Work out the finished part from the listing and answer in its coordinate system (mm). A direction names the side the tool comes from. Round coordinates to 2 decimals unless told otherwise and drop trailing zeros. Loops run counter-clockwise (first coordinate to the right, second up) from the corner with the lowest first, then second, coordinate; pieces in that order, holes last. Notation, with made-up numbers: (-17.5, 61) -> (40.5, 61) arc R6 cw to (40.5, 66) -> close; hole circle Ø10 at (6, 41.25). An arc over 180 degrees is marked (long way). Use one line per item in the form item = value.
```python
from build123d import *

# Parameters (mm, degrees)
F0_R     = 10
F0_R_2   = 6.25
F1_DEPTH = 5
F0_R_3   = 5
F2_DEPTH = 55
F3_DEPTH = 51


# Not quite as in the source:
# - a fillet or chamfer that OpenCascade refuses, or shapes differently, is made with other operations: its cross-section is extruded or revolved along the edge and cut away or added


with BuildPart() as f1:
    # F0 (on Top) → F1 (new body)
    with BuildSketch(Plane.XY):
        Circle(F0_R)
        Circle(F0_R_2, mode=Mode.SUBTRACT)
    extrude(amount=F1_DEPTH)

    # F0 (on Top) → F2 (join)
    with BuildSketch(Plane.XY):
        Circle(F0_R_2)
        Circle(F0_R_3, mode=Mode.SUBTRACT)
    extrude(amount=F2_DEPTH)

    # F0 (on Top) → F3 (cut)
    with BuildSketch(Plane.XY):
        Circle(F0_R_3)
    extrude(amount=F3_DEPTH, mode=Mode.SUBTRACT)

    # F4: fillet of radius 2 on 3 edges, made by hand

    # F4_s1 → F4_t2 (revolve, cut)
    with BuildSketch(Plane.XZ):
        with BuildLine():
            ThreePointArc((5, 2), (5.5857864376, 0.5857864376), (7, 0))
            Line((7, 0), (5, 0))
            Line((5, 0), (5, 2))
        make_face()
    revolve(axis=Axis((0, 0, 0), (0, 0, 1)), mode=Mode.SUBTRACT)

    # F4_s3 → F4_t4 (revolve, cut)
    with BuildSketch(Plane.XZ):
        with BuildLine():
            ThreePointArc((6.25, 55), (5.3416876048, 54.263984367), (5, 53.1459503782))
            Line((5, 53.1459503782), (5, 55))
            Line((5, 55), (6.25, 55))
        make_face()
    revolve(axis=Axis((0, 0, 55), (0, 0, 1)), mode=Mode.SUBTRACT)

    # F4_s5 → F4_t6 (revolve, cut)
    with BuildSketch(Plane.XZ):
        with BuildLine():
            ThreePointArc((10, 2), (9.4142135624, 0.5857864376), (8, 0))
            Line((8, 0), (10, 0))
            Line((10, 0), (10, 2))
        make_face()
    revolve(axis=Axis((0, 0, 0), (0, 0, 1)), mode=Mode.SUBTRACT)


solid = f1.part
```
(1) For a pull along Y with two mould halves and no side action, classify faces 1 (the cylindrical face through (-1.08, -4.88, 27.21)), 2 (the cylindrical face through (5.96, 1.88, 29.65)), 3 (the flat face through (4, -6, 0)) as +Y half, -Y half, draft (parallel to the pull), parting line (faces both ways), or undercut.
Completed:
face_1 = undercut
face_2 = parting line
face_3 = draft
(2) Consider L1, parallel to Y at x = 0, z = 41; L2, parallel to Y at x = -3.5, z = 52; L3, parallel to Z at x = -7.5, y = 2. Determine where each line is inside the solid, lowest interval first.
Completed:
L1 = -6.25 to -5, 5 to 6.25
L2 = -5.18 to -3.57, 3.57 to 5.18
L3 = 0 to 5
(3) Given P1, Ø10, axis at y = 5, z = 24, coming from the -X side; P2, Ø8, axis at y = -3.5, z = 26.5, coming from the +X side; P3, Ø10, axis at x = -1.5, y = 0.5, coming from the +Z side; P4, Ø3, axis at x = 6.5, z = 47.5, coming from the +Y side, each flat-ended and moving along its own axis, determine where each tip first touches the part or whether it passes through.
Completed:
P1 = -6.25
P2 = 6.25
P3 = 55
P4 = 3.75
(4) For faces 4 (the flat face through (4, 5, 5)), 5 (the cylindrical face through (-2.17, -9.76, 3.48)), determine the directions among +Z, -Z, +X, -X, +Y, -Y from which every point of the face is accessible in a straight line to the end or side of a thin tool.
Completed:
face_4 = +Z
face_5 = +Z, -Z
(5) Find section A-A, the plane y = 0. Write down the section's boundary in (x, z), then the cut area to 3 significant figures.
Completed:
outline = (-10, 2) arc R2 ccw to (-8, 0) -> (-7, 0) arc R2 ccw to (-5, 2) -> (-5, 53.15) arc R2 ccw to (-6.25, 55) -> (-6.25, 5) -> (-10, 5) -> close; (5, 2) arc R2 ccw to (7, 0) -> (8, 0) arc R2 ccw to (10, 2) -> (10, 5) -> (6.25, 5) -> (6.25, 55) arc R2 ccw to (5, 53.15) -> close
area = 170 mm2
(6) Find section C-C, the plane z = 24. Write down the section's boundary in (x, y), then the cut area to 3 significant figures.
Completed:
outline = circle Ø12.5 at (0, 0); hole circle Ø10 at (0, 0)
area = 44.2 mm2
